```python
from build123d import *

# Parameters (mm, degrees)
F1_DEPTH = 50
F3_DEPTH = 350
F4_R     = 5


with BuildPart() as f1:
    # F0 (on Top) → F1 (new body)
    with BuildSketch(Plane.XY):
        with BuildLine():
            Line((153.906826, 208.065538), (-186.093174, 208.065538))
            ThreePointArc((-186.093174, 208.065538), (-207.306378, 199.278742), (-216.093174, 178.065538))
            Line((-216.093174, 178.065538), (-216.093174, -161.934462))
            ThreePointArc((-216.093174, -161.934462), (-207.306378, -183.147665), (-186.093174, -191.934462))
            Line((-186.093174, -191.934462), (153.906826, -191.934462))
            ThreePointArc((153.906826, -191.934462), (175.120029, -183.147665), (183.906826, -161.934462))
            Line((183.906826, -161.934462), (183.906826, 178.065538))
            ThreePointArc((183.906826, 178.065538), (175.120029, 199.278742), (153.906826, 208.065538))
        make_face()
    extrude(amount=F1_DEPTH)

    # F2 (on Top) → F3 (join)
    with BuildSketch(Plane.XY):
        with BuildLine():
            Line((113.906826, -151.934462), (133.906826, -151.934462))
            ThreePointArc((133.906826, -151.934462), (140.977893, -149.005529), (143.906826, -141.934462))
            Line((143.906826, -141.934462), (143.906826, -121.934462))
            ThreePointArc((143.906826, -121.934462), (140.977893, -114.863394), (133.906826, -111.934462))
            Line((133.906826, -111.934462), (113.906826, -111.934462))
            ThreePointArc((113.906826, -111.934462), (106.835758, -114.863394), (103.906826, -121.934462))
            Line((103.906826, -121.934462), (103.906826, -141.934462))
            ThreePointArc((103.906826, -141.934462), (106.835758, -149.005529), (113.906826, -151.934462))
        make_face()
        with BuildLine():
            Line((113.906826, 128.065538), (133.906826, 128.065538))
            ThreePointArc((133.906826, 128.065538), (140.977893, 130.994471), (143.906826, 138.065538))
            Line((143.906826, 138.065538), (143.906826, 158.065538))
            ThreePointArc((143.906826, 158.065538), (140.977893, 165.136606), (133.906826, 168.065538))
            Line((133.906826, 168.065538), (113.906826, 168.065538))
            ThreePointArc((113.906826, 168.065538), (106.835758, 165.136606), (103.906826, 158.065538))
            Line((103.906826, 158.065538), (103.906826, 138.065538))
            ThreePointArc((103.906826, 138.065538), (106.835758, 130.994471), (113.906826, 128.065538))
        make_face()
        with BuildLine():
            Line((-166.093174, 128.065538), (-146.093174, 128.065538))
            ThreePointArc((-146.093174, 128.065538), (-139.022107, 130.994471), (-136.093174, 138.065538))
            Line((-136.093174, 138.065538), (-136.093174, 158.065538))
            ThreePointArc((-136.093174, 158.065538), (-139.022107, 165.136606), (-146.093174, 168.065538))
            Line((-146.093174, 168.065538), (-166.093174, 168.065538))
            ThreePointArc((-166.093174, 168.065538), (-173.164242, 165.136606), (-176.093174, 158.065538))
            Line((-176.093174, 158.065538), (-176.093174, 138.065538))
            ThreePointArc((-176.093174, 138.065538), (-173.164242, 130.994471), (-166.093174, 128.065538))
        make_face()
        with BuildLine():
            Line((-166.093174, -151.934462), (-146.093174, -151.934462))
            ThreePointArc((-146.093174, -151.934462), (-139.022107, -149.005529), (-136.093174, -141.934462))
            Line((-136.093174, -141.934462), (-136.093174, -121.934462))
            ThreePointArc((-136.093174, -121.934462), (-139.022107, -114.863394), (-146.093174, -111.934462))
            Line((-146.093174, -111.934462), (-166.093174, -111.934462))
            ThreePointArc((-166.093174, -111.934462), (-173.164242, -114.863394), (-176.093174, -121.934462))
            Line((-176.093174, -121.934462), (-176.093174, -141.934462))
            ThreePointArc((-176.093174, -141.934462), (-173.164242, -149.005529), (-166.093174, -151.934462))
        make_face()
    extrude(amount=F3_DEPTH)

    # F4
    f4_edges = [f1.edges().sort_by_distance(p)[0] for p in [
        (-16.093174, 208.065538, 0),
    ]]
    fillet(f4_edges, radius=F4_R)


solid = f1.part
```
The listing builds one solid part. Answer for the finished solid, in the listing's coordinates (mm). A direction names the side the tool comes from. Round coordinates to 2 decimals unless told otherwise and drop trailing zeros. Loops run counter-clockwise (first coordinate to the right, second up) from the corner with the lowest first, then second, coordinate; pieces in that order, holes last.
Q1. Given pin 1 Ø22 at (y, z) = (-128, 142) entering from -X; pin 2 Ø10 at (x, z) = (128, 188) entering from -Y; pin 3 Ø1 at (y, z) = (130, 102) entering from -X, each flat-ended and moving along its own axis, determine where each tip first touches the part or whether it passes through.
Q2. Section C-C, the plane y = 31.5 is taken. Determine the outline of the cut face in (x, z), then the cut area to 3 significant figures.
Q3. Section A-A, the plane z = 210.5 is taken. Count the separate pieces of the cut face and the enclosed holes in it, then the cut area to 3 significant figures.
Q4. Find the intervals of material crossed by line 1 (X direction, y = 142.5, z = 136); line 2 (Y direction, x = 135.5, z = 305.5); line 3 (Z direction, x = 138.5, y = 66.5), in increasing order.
Q5. Section B-B, the plane x = 122.5 is taken. Determine the outline of the cut face in (y, z).
Q6. For a pull along Y with two mould halves and no side action, classify faces 1 (the face through (143.907, -132, 198)), 2 (the face through (106.76, 131.07, 197.9)), 3 (the face through (-207.54, -182.91, 27.18)) as released by +Y, released by -Y, zero draft, split by the parting line, or undercut.
Q7. Which of the six approach directions +Z, -Z, +X, -X, +Y, -Y give full straight-line access (tool end or side, diameter ignored) to faces 4 (the face through (141.055, -114.942, 197.9)), 5 (the face through (-136.093, -132, 198)), 6 (the face through (124, 128.066, 198))?
Q8. Section D-D, the plane x = -122.5 is taken. Determine the outline of the cut face in (y, z), then the cut area to 3 significant figures.
Completed:
1. pin 1: stops at x = -176.09
1. pin 2: stops at y = -151.93
1. pin 3: stops at x = -172.63
2. outline: (-216.09, 5) arc R5 ccw to (-211.09, 0) - (178.91, 0) arc R5 ccw to (183.91, 5) - (183.91, 50) - (-216.09, 50) - close
2. area: 20,000 mm2
3. separate pieces: 4
3. enclosed holes: 0
3. area: 6,060 mm2
4. line 1: x = -176.09 to -136.09, 103.91 to 143.91
4. line 2: y = -151.81 to -112.06, 128.19 to 167.94
4. line 3: z = 0 to 50
5. outline: (-191.93, 5) arc R5 ccw to (-186.93, 0) - (203.07, 0) arc R5 ccw to (208.07, 5) - (208.07, 50) - (168.07, 50) - (168.07, 350) - (128.07, 350) - (128.07, 50) - (-111.93, 50) - (-111.93, 350) - (-151.93, 350) - (-151.93, 50) - (-191.93, 50) - close
6. face 1: zero draft
6. face 2: undercut
6. face 3: released by -Y
7. face 4: +Z, +X
7. face 5: +Z, +Y, -Y
7. face 6: +Z, +X, -X
8. outline: (-191.93, 5) arc R5 ccw to (-186.93, 0) - (203.07, 0) arc R5 ccw to (208.07, 5) - (208.07, 50) - (-191.93, 50) - close
8. area: 20,000 mm2
